from build123d import *

# Parameters (mm, degrees)
F0_R     = 15.875
F1_DEPTH = 2
F2_W     = 20.42
F2_H     = 13.35
F3_DEPTH = 2
F4_R     = 5.26728
F5_DEPTH = 5


with BuildPart() as f1:
    # F0 (on Top) → F1 (new body)
    with BuildSketch(Plane.XY):
        Circle(F0_R)
    extrude(amount=F1_DEPTH)

    # F2 (on face) → F3 (cut)
    with BuildSketch(Plane.XY.offset(2)):
        with Locations((-0.826221, 0.604355)):
            Rectangle(F2_W, F2_H)
    extrude(amount=-F3_DEPTH, mode=Mode.SUBTRACT)

    # F4 (on face) → F5 (cut)
    with BuildSketch(Plane.XY.offset(2)):
        with Locations((16.107954, -9.460228)):
            Circle(F4_R)
    extrude(amount=-F5_DEPTH, mode=Mode.SUBTRACT)


solid = f1.part
Input: part model. Units: mm. Frame: model coordinates. A direction names the side the tool comes from. Coordinates: 2 decimals unless noted, no trailing zeros. Loops run counter-clockwise (first coordinate to the right, second up) from the corner with the lowest first, then second, coordinate; pieces in that order, holes last.
(1) Section D-D on y = -9. Return the cut outline in (x, z).
(2) Section B-B on x = 0. Return the cut outline in (y, z) (3 decimals), then the cut area to 3 significant figures.
(3) Pull-direction query (X, two-part tool) for faces 1 (the face through (-11.036, 1, 1)), 2 (the face through (11.599, -6.737, 1.014)), 3 (the face through (0, -7, 2)); classes: released by +X, released by -X, zero draft, split by the parting line, or undercut.
(4) Section C-C on z = 0.85. Return the cut outline in (x, y) (3 decimals).
(5) Section A-A on y = 0. Return the cut outline in (x, z) (3 decimals), then the cut area to 3 significant figures.
(6) Set-up query: faces 4 (the face through (-1, -6.071, 1)), 5 (the face through (0, -7, 0)). Return all of +Z, -Z, +X, -X, +Y, -Y with unobstructed straight access to the full face (end or side cutting, diameter ignored); none if empty.
(7) First-contact query: pin 1 Ø1 at (y, z) = (9.5, 1) entering from -X. Flat tip, straight axial feed; report the tip coordinate or a pass-through.
(8) Material intervals for probe 1 along X at (y, z) = (1, 1.55); probe 2 along Y at (x, z) = (1.5, 0.1); probe 3 along Y at (x, z) = (4.5, 1.45), sorted ascending.
Data:
1. outline: (-13.08, 0) - (10.86, 0) - (10.86, 2) - (-13.08, 2) - close
2. outline: (-15.875, 0) - (-6.071, 0) - (-6.071, 2) - (-15.875, 2) - close; (7.279, 0) - (15.875, 0) - (15.875, 2) - (7.279, 2) - close
2. area: 36.8 mm2
3. face 1: undercut
3. face 2: released by +X
3. face 3: zero draft
4. outline: (11.166, -11.284) arc R5.267 cw to (15.294, -4.256) arc R15.875 ccw (long way) to start; hole (-11.036, -6.071) - (9.384, -6.071) - (9.384, 7.279) - (-11.036, 7.279) - close
5. outline: (-15.875, 0) - (-11.036, 0) - (-11.036, 2) - (-15.875, 2) - close; (9.384, 0) - (15.875, 0) - (15.875, 2) - (9.384, 2) - close
5. area: 22.7 mm2
6. face 4: +Z, -Z
6. face 5: -Z, +X, -X, +Y, -Y
7. pin 1: stops at x = -13.08
8. probe 1: x = -15.84 to -11.04, 9.38 to 15.84
8. probe 2: y = -15.8 to -6.07, 7.28 to 15.8
8. probe 3: y = -15.22 to -6.07, 7.28 to 15.22
